```python
from build123d import *

# Parameters (mm, degrees)
F1_DEPTH = 5
F2_DEPTH = 2
F3_DEPTH = 2
F4_R     = 1
F5_D     = 2


with BuildPart() as f1:
    # F0 (on Top) → F1 (new body)
    with BuildSketch(Plane.XY):
        with BuildLine():
            ThreePointArc((-6.139429, -0.003584), (-6.139428, -0.001792), (-6.139428, 0))
            ThreePointArc((-6.139428, 0), (-16.03356, 1.023463), (-6.558418, -2.003584))
            ThreePointArc((-6.558418, -2.003584), (-6.245664, -1.025217), (-6.139429, -0.003584))
        make_face()
    extrude(amount=-F1_DEPTH)

    # F0 (on Top) → F2 (join)
    with BuildSketch(Plane.XY):
        with BuildLine():
            ThreePointArc((-6.139429, -0.003584), (-6.245664, -1.025217), (-6.558418, -2.003584))
            Line((-6.558418, -2.003584), (-1.139429, -2.003584))
            Line((-1.139429, -2.003584), (-1.139429, -0.003584))
            Line((-1.139429, -0.003584), (-6.139429, -0.003584))
        make_face()
    extrude(amount=-F2_DEPTH)

    # F0 (on Top) → F3 (join, symmetric)
    with BuildSketch(Plane.XY):
        Polygon((-1.139429, -0.003584), (-1.139429, -2.003584), (-1.139429, -4.003584), (4.056571, -1.003584), (4.056571, -0.003584), align=None)
    extrude(amount=F3_DEPTH, both=True)

    # F4
    f4_edges = [f1.edges().sort_by_distance(p)[0] for p in [
        (-1.139429, -4.003584, 0),
    ]]
    fillet(f4_edges, radius=F4_R)

    # F5 (through all)
    with Locations(Plane.XY):
        with Locations((-11.139428, 0)):
            Hole(F5_D / 2)


solid = f1.part
```
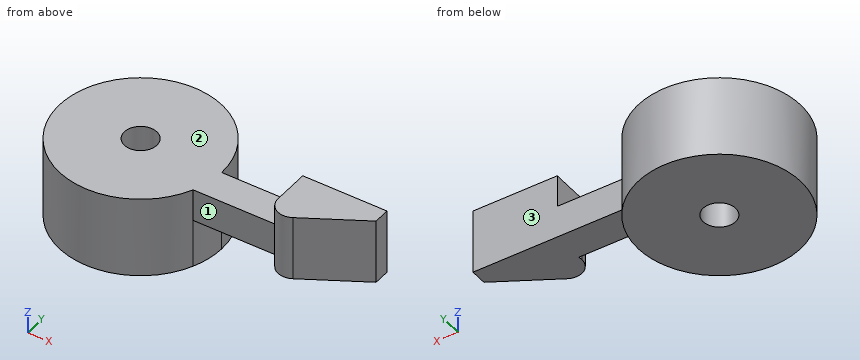
Could you check a few things on this model? Use its own coordinates, in mm. Face numbers are marked on the shaded views. A direction names the side the tool comes from. Coordinates: 2 decimals unless noted, no trailing zeros. Write each loop counter-clockwise with the first axis right and the second up, starting at its lowest first coordinate (ties: lowest second). Pieces come first, ordered by that corner, then holes. Notation, with made-up numbers: M 44.25,8 L 87.25,8 A32 cw 87.25,47 Z; hole C -21,43 d2. An arc over 180 degrees is marked long. Answer as CSV lines item,"result". Start each with the question number.
1) I want a section at C-C, the plane y = 0.75. Please give me the cut outline in (x, z).
2) For the marked faces 1, 2 and 3, which set-ups out of +Z, -Z, +X, -X, +Y, -Y let a thin tool reach every point of the face, with its end or its side?
3) I want a section at B-B, the plane x = -11.75. Please give me the cut outline in (y, z), and give its area (3 significant figures).
4) Please list where these lines run through material, in increasing order: line 1 (Z direction, x = -1.75, y = -1.5); line 2 (Z direction, x = -10, y = 2.25); line 3 (Y direction, x = 1.75, z = -1.5). Write a range as from..to.
5) I want a section at D-D, the plane y = -1.25. Please give me the cut outline in (x, z), and give its area (3 significant figures).
6) For P1, Ø1, axis at x = -4, z = -1.5, coming from the -Y side; P2, Ø1.6, axis at x = -2, y = -1, coming from the -Z side; P3, Ø1.5, axis at x = -2.5, z = -3, coming from the -Y side; P4, Ø4, axis at x = -7, z = -2.5, coming from the +Y side, each with a flat end and sliding along its axis, tell me the tip position at first contact or that it passes through.
Data:
1,outline,"M -16.08,-5 L -11.8,-5 L -11.8,0 L -16.08,0 Z; M -10.48,-5 L -6.2,-5 L -6.2,0 L -10.48,0 Z"
2,face 1,"+Z, -Z, -Y"
2,face 2,"+Z, -X, +Y, -Y"
2,face 3,"+Z, -Z, +X, +Y"
3,outline,"M -4.96,-5 L -0.79,-5 L -0.79,0 L -4.96,0 Z; M 0.79,-5 L 4.96,-5 L 4.96,0 L 0.79,0 Z"
3,area,"41.7 mm^2"
4,line 1,"z = -2..0"
4,line 2,"z = -5..0"
4,line 3,"y = -2.34..0"
5,outline,"M -15.98,-5 L -6.3,-5 L -6.3,-2 L 3.63,-2 L 3.63,2 L -1.14,2 L -1.14,0 L -15.98,0 Z"
5,area,"77.8 mm^2"
6,P1,"stops at y = -2"
6,P2,"stops at z = -2"
6,P3,"passes through"
6,P4,"stops at y = 4.52"
